Geometry check sheet. Reference: the model listing, model coordinates, mm. A direction names the side the tool comes from. Round coordinates to 2 decimals unless told otherwise and drop trailing zeros. Write each loop counter-clockwise with the first axis right and the second up, starting at its lowest first coordinate (ties: lowest second). Pieces come first, ordered by that corner, then holes. Notation, with made-up numbers: (56.5, -11) - (101.5, -11) arc R19 ccw to (101.5, 14) - close; hole circle Ø11 at (1, -39.5). An arc over 180 degrees is marked (long way). Return JSON: item names as keys, results as strings. Group by question number.
from build123d import *

# Parameters (mm, degrees)
ESQUISSE1_W                = 40
ESQUISSE1_H                = 10
BOSS_EXTRU_1_DEPTH         = 3
ESQUISSE2_W                = 40
ESQUISSE2_H                = 2.9
BOSS_EXTRU_2_DEPTH         = 1
ESQUISSE3_R                = 1.5
ENL_V_MAT_EXTRU_1_DEPTH    = 5
R_P_TITION_LIN_AIRE1_COUNT = 4
R_P_TITION_LIN_AIRE1_PITCH = 10


with BuildPart() as part:
    # Esquisse1 → Boss.-Extru.1 (new body)
    with BuildSketch(Plane.XY):
        with Locations((20, 5)):
            Rectangle(ESQUISSE1_W, ESQUISSE1_H)
    extrude(amount=BOSS_EXTRU_1_DEPTH)

    # Esquisse2 → Boss.-Extru.2 (add)
    with BuildSketch(Plane.XY.offset(3)):
        with Locations((20, 5)):
            Rectangle(ESQUISSE2_W, ESQUISSE2_H)
    extrude(amount=BOSS_EXTRU_2_DEPTH)

    # Esquisse3 → Enlèv. mat.-Extru.1 (cut, through all)
    with BuildSketch(Plane(origin=(0, 0, 0), x_dir=(-1, 0, 0), z_dir=(0, 0, -1))):
        with Locations((-35, 5)):
            Circle(ESQUISSE3_R)
    enl_v_mat_extru_1 = extrude(amount=-ENL_V_MAT_EXTRU_1_DEPTH, mode=Mode.SUBTRACT)

    # Répétition linéaire1: Enlèv. mat.-Extru.1 ×4
    with Locations(*[(-i * R_P_TITION_LIN_AIRE1_PITCH, 0, 0) for i in range(1, R_P_TITION_LIN_AIRE1_COUNT)]):
        add(enl_v_mat_extru_1, mode=Mode.SUBTRACT)


solid = part.part
1. Material ranges on line 1 along Y through (x, z) = (5, 2.9); line 2 along X through (y, z) = (6, 2.35); line 3 along X through (y, z) = (4.5, 3.3), recorded low to high.
2. Section check C-C (y = 2.75). Enter the section's corners in (x, z), and give its area (3 significant figures).
3. Depth check by flat-ended pin: pin 1 Ø1.1 at (x, y) = (11.5, 9) entering from +Z; pin 2 Ø0.5 at (x, z) = (3.5, 3.5) entering from +Y; pin 3 Ø0.5 at (x, z) = (30.5, 3.5) entering from -Y. Enter the tip coordinate at first touch or a pass-through.
4. Section check B-B (z = 0.6). Enter the section's corners in (x, y).
5. Tool access check on faces 1 (the face through (23.57, 5.45, 1.97)), 2 (the face through (37.7, 6.45, 3.5)), 3 (the face through (9.9, 3.55, 3.5)). Record the directions out of +Z, -Z, +X, -X, +Y, -Y that give a thin tool (end or side, any length) a straight path to the whole face; none if there is none.
6. Section check A-A (x = 5). Enter the section's corners in (y, z).
7. Mould release check, pull along Y, two halves, no side actions. Record for faces 4 (the face through (2.3, 6.45, 3.5)), 5 (the face through (20, 5, 0)), 6 (the face through (3.57, 5.45, 1.97)): pulls with the +Y half, pulls with the -Y half, needs draft (parallel to the pull), parting line crosses it, or undercut.
Result sheet:
{
 "1": {"line 1": "y = 0 to 3.5, 6.5 to 10", "line 2": "x = 0 to 3.88, 6.12 to 13.88, 16.12 to 23.88, 26.12 to 33.88, 36.12 to 40", "line 3": "x = 0 to 3.59, 6.41 to 13.59, 16.41 to 23.59, 26.41 to 33.59, 36.41 to 40"},
 "2": {"outline": "(0, 0) - (40, 0) - (40, 3) - (0, 3) - close", "area": "120 mm²"},
 "3": {"pin 1": "stops at z = 3", "pin 2": "stops at y = 6.45", "pin 3": "stops at y = 3.55"},
 "4": {"outline": "(0, 0) - (40, 0) - (40, 10) - (0, 10) - close; hole circle Ø3 at (5, 5); hole circle Ø3 at (15, 5); hole circle Ø3 at (25, 5); hole circle Ø3 at (35, 5)"},
 "5": {"face 1": "+Z, -Z", "face 2": "+Z, +X, -X, +Y", "face 3": "+Z, +X, -X, -Y"},
 "6": {"outline": "(0, 0) - (3.5, 0) - (3.5, 3) - (0, 3) - close; (6.5, 0) - (10, 0) - (10, 3) - (6.5, 3) - close"},
 "7": {"face 4": "pulls with the +Y half", "face 5": "needs draft", "face 6": "undercut"}
}
